Here's how the part is built. I have some questions about the finished solid (model axes, mm). Face numbers are marked on the shaded views. Coordinates: 2 decimals unless noted, no trailing zeros. Order: outer loops, then holes, each group sorted by start corner. A loop starts at its lowest first (then second) coordinate and runs counter-clockwise, first axis right, second up. Notation, with made-up numbers: (12.5, -23.75) -> (64.5, -23.75) arc R20 cw to (64.5, 9.25) -> close; hole circle Ø3 at (-27.5, 65). An arc over 180 degrees is marked (long way). One line per item, written item: value. Start each with the question number.
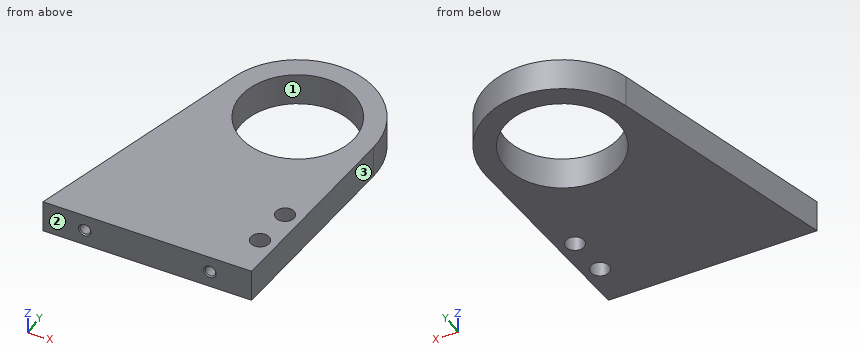
```python
from build123d import *

# Parameters (mm, degrees)
SKETCH_1_R                   = 19
SKETCH_1_R_2                 = 14
EXTRUDE_1_DEPTH              = 8
HOLE_WIZARD_M4_1_D           = 4.5
HOLE_WIZARD_M3_1_D           = 2.5
HOLE_WIZARD_M3_1_DEPTH       = 8.5
HOLE_WIZARD_M3_1_CSINK_D     = 3.05
HOLE_WIZARD_M3_1_CSINK_ANGLE = 90
HOLE_WIZARD_M3_1_TIP         = 0.751075774


with BuildPart() as part:
    # 스케치1 → 보스-돌출1 (new body)
    # profile 1 of 2: a face of its own
    with BuildSketch(Plane.XY):
        with BuildLine():
            Line((16.816107383, 55.508724832), (0, 0))
            Line((0, 0), (50, 0))
            Line((50, 0), (53.937590447, 48.461277134))
            ThreePointArc((53.937590447, 48.461277134), (31.456182162, 31.333416083), (16.816107383, 55.508724832))
        make_face()
    # profile 2 of 2: a face of its own
    with BuildSketch(Plane.XY):
        with Locations((35, 50)):
            Circle(SKETCH_1_R)
        with Locations((35, 50)):
            Circle(SKETCH_1_R_2, mode=Mode.SUBTRACT)
    extrude(amount=EXTRUDE_1_DEPTH)

    # M4 여유 구멍1 (through all)
    with Locations(Plane.XY.offset(8)):
        with Locations((46.799340892, 10), (47.609195032, 19.967152867)):
            Hole(HOLE_WIZARD_M4_1_D / 2)

    # M3 나사 구멍1
    with Locations(Plane(origin=(0, 0, 0), x_dir=(-1, 0, 0), z_dir=(0, -1, 0))):
        with Locations((-10, -4), (-40, -4)):
            CounterSinkHole(HOLE_WIZARD_M3_1_D / 2, HOLE_WIZARD_M3_1_CSINK_D / 2, depth=HOLE_WIZARD_M3_1_DEPTH, counter_sink_angle=HOLE_WIZARD_M3_1_CSINK_ANGLE)
            with Locations((0, 0, -(HOLE_WIZARD_M3_1_DEPTH + HOLE_WIZARD_M3_1_TIP / 2))):  # 118° drill point
                Cone(0, HOLE_WIZARD_M3_1_D / 2, HOLE_WIZARD_M3_1_TIP, mode=Mode.SUBTRACT)


solid = part.part
```
Q1. For P1, Ø1, axis at y = 43.5, z = 4.5, coming from the +X side; P2, Ø4, axis at x = 14, y = 54, coming from the -Z side; P3, Ø1.5, axis at x = 40, z = 4, coming from the -Y side; P4, Ø2, axis at x = 10, z = 4, coming from the -Y side, each with a flat end and sliding along its axis, tell me the tip position at first contact or that it passes through.
Q2. Imagine slicing it at A-A (x = 35). Write out the boundary of the cut face in (y, z).
Q3. Imagine slicing it at B-B (y = 50). Write out the boundary of the cut face in (x, z), plus the area to 3 significant figures.
Q4. Imagine slicing it at C-C (x = 47.5). Write out the boundary of the cut face in (y, z), plus the area to 3 significant figures.
Q5. Imagine slicing it at D-D (z = 1.75). Write out the boundary of the cut face in (x, y), plus the area to 3 significant figures.
Q6. If we mould it in two halves opening along X, with no side actions, what happens to the marked faces 1, 2 and 3? For each: +X half, -X half, draft (parallel to the pull), parting line (faces both ways), or undercut.
Q7. I need wall thicknesses on line 1 (Z direction, x = 10, y = 5); line 2 (Y direction, x = 35, z = 4.25); line 3 (X direction, y = 4.75, z = 4). Which ranges of each line are inside material? Lowest first, please.
Completed:
1. P1: stops at x = 53.58
1. P2: passes through
1. P3: stops at y = 8.8
1. P4: stops at y = 8.65
2. outline: (0, 0) -> (36, 0) -> (36, 8) -> (0, 8) -> close; (64, 0) -> (69, 0) -> (69, 8) -> (64, 8) -> close
3. outline: (15.15, 0) -> (21, 0) -> (21, 8) -> (15.15, 8) -> close; (49, 0) -> (54, 0) -> (54, 8) -> (49, 8) -> close
3. area: 86.8 mm2
4. outline: (0, 0) -> (7.86, 0) -> (7.86, 8) -> (0, 8) -> close; (12.14, 0) -> (17.72, 0) -> (17.72, 8) -> (12.14, 8) -> close; (22.21, 0) -> (43.7, 0) -> (43.7, 8) -> (22.21, 8) -> close; (56.3, 0) -> (64.31, 0) -> (64.31, 8) -> (56.3, 8) -> close
4. area: 343 mm2
5. outline: (0, 0) -> (50, 0) -> (53.94, 48.46) arc R19 ccw to (16.82, 55.51) -> close; hole circle Ø28 at (35, 50); hole circle Ø4.5 at (46.8, 10); hole circle Ø4.5 at (47.61, 19.97)
5. area: 2,140 mm2
6. face 1: undercut
6. face 2: draft
6. face 3: +X half
7. line 1: z = 0 to 2.75, 5.25 to 8
7. line 2: y = 0 to 36, 64 to 69
7. line 3: x = 1.44 to 8.75, 11.25 to 38.75, 41.25 to 50.39
